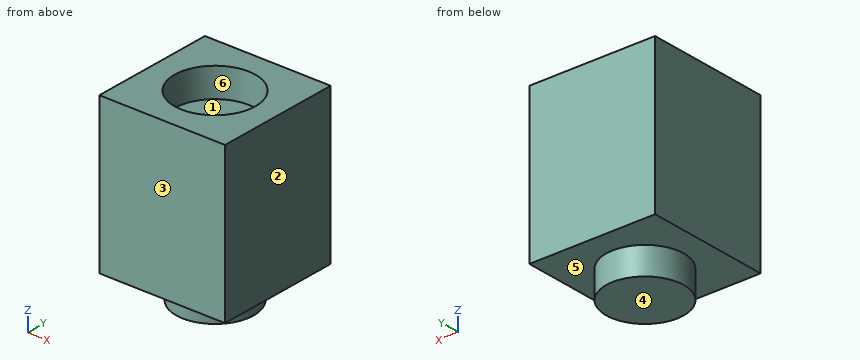
from build123d import *

# Parameters (mm, degrees)
SKETCH_1_W          = 7.8
SKETCH_1_H          = 7.8
EXTRUDE_1_DEPTH     = 9.6
SKETCH_2_R          = 2.4
EXTRUDE_2_DEPTH     = 1.7
SKETCH_3_R          = 2.5
CUT_EXTRUDE_1_DEPTH = 1.8


with BuildPart() as part:
    # Эскиз1 → Бобышка-Вытянуть1 (new body)
    with BuildSketch(Plane.XY):
        Rectangle(SKETCH_1_W, SKETCH_1_H)
    extrude(amount=EXTRUDE_1_DEPTH)

    # Эскиз2 → Бобышка-Вытянуть2 (add)
    with BuildSketch(Plane(origin=(0, 0, 0), x_dir=(-1, 0, 0), z_dir=(0, 0, -1))):
        Circle(SKETCH_2_R)
    extrude(amount=EXTRUDE_2_DEPTH)

    # Эскиз3 → Вырез-Вытянуть1 (cut)
    with BuildSketch(Plane.XY.offset(9.6)):
        Circle(SKETCH_3_R)
    extrude(amount=-CUT_EXTRUDE_1_DEPTH, mode=Mode.SUBTRACT)


solid = part.part
Verification items for the finished model (mm, model axes). Face numbers are marked on the shaded views. A direction names the side the tool comes from. Coordinates: 2 decimals unless noted, no trailing zeros. Order: outer loops, then holes, each group sorted by start corner. A loop starts at its lowest first (then second) coordinate and runs counter-clockwise, first axis right, second up. Notation, with made-up numbers: (-3, 42) -> (34, 42) arc R3 cw to (34, 46) -> close; hole circle Ø4 at (12, 55.25). An arc over 180 degrees is marked (long way). Put each result on its own line as item: value. Start each with the question number.
1. Cross-section at A-A, the plane y = 0. Record the boundary of the cut face in (x, z), then the cut area to 3 significant figures.
2. Mould release check, pull along X, two halves, no side actions. Record for the marked faces 1, 2 and 3: released by +X, released by -X, zero draft, split by the parting line, or undercut.
3. Cross-section at C-C, the plane y = 3.25. Record the boundary of the cut face in (x, z).
4. Material ranges on L1, parallel to Y at x = 0, z = 8.9; L2, parallel to Z at x = 1.5, y = 0; L3, parallel to Z at x = 1.5, y = -2.5, recorded low to high. Write a range as [from, to].
5. Access from +Z, -Z, +X, -X, +Y, -Y to the whole of each face (thin tool, end or side, straight path). Record for the marked faces 4, 5 and 6.
Computed:
1. outline: (-3.9, 0) -> (-2.4, 0) -> (-2.4, -1.7) -> (2.4, -1.7) -> (2.4, 0) -> (3.9, 0) -> (3.9, 9.6) -> (2.5, 9.6) -> (2.5, 7.8) -> (-2.5, 7.8) -> (-2.5, 9.6) -> (-3.9, 9.6) -> close
1. area: 74.0 mm2
2. face 1: undercut
2. face 2: released by +X
2. face 3: zero draft
3. outline: (-3.9, 0) -> (3.9, 0) -> (3.9, 9.6) -> (-3.9, 9.6) -> close
4. L1: [-3.9, -2.5], [2.5, 3.9]
4. L2: [-1.7, 7.8]
4. L3: [0, 9.6]
5. face 4: -Z, +X, -X, +Y, -Y
5. face 5: -Z
5. face 6: +Z
